Geometry check sheet. Reference: the model listing, model coordinates, mm. A direction names the side the tool comes from. Give positions to 0.01 mm unless a question says otherwise; leave off trailing zeros. Loops run counter-clockwise (first coordinate to the right, second up) from the corner with the lowest first, then second, coordinate; pieces in that order, holes last. Notation, with made-up numbers: (-35.75, 20) - (-28.75, 20) arc R11 ccw to (-28.75, 37) - close; hole circle Ø10 at (5.25, 63). An arc over 180 degrees is marked (long way). Use a Markdown table: item, result. Add a question column.
1. Depth check by flat-ended pin: P1, Ø2.5, axis at x = -16.5, y = -30, coming from the +Z side; P2, Ø6, axis at x = -47.5, y = 0, coming from the -Z side; P3, Ø1, axis at y = -22.5, z = 1, coming from the +X side. Enter the tip coordinate at first touch or a pass-through.
2. Cross-section at B-B on y = -37.5. Enter the section's corners in (x, z), and give its area (3 significant figures).
3. Material ranges on L1, parallel to X at y = -2, z = 1.8; L2, parallel to X at y = 29.5, z = 1.7; L3, parallel to Y at x = 0, z = 1.6, recorded low to high.
4. Cross-section at A-A on x = 47.5. Enter the section's corners in (y, z), and give its area (3 significant figures).
5. Cross-section at C-C on y = -20. Enter the section's corners in (x, z), and give its area (3 significant figures).
6. Draft check along Y on faces 1 (the flat face through (17, -31, 2)), 2 (the cylindrical face through (-11.923, -53.692, 1.479)), 3 (the flat face through (-1, 1, 0)). Enter one of: pulls with the +Y half, pulls with the -Y half, needs draft (parallel to the pull), parting line crosses it, or undercut.
7. Set-up check for faces 4 (the cylindrical face through (45.19, -0.96, 1.48)), 5 (the flat face through (-34, -2, 2)): record each of +Z, -Z, +X, -X, +Y, -Y from which the full face is reachable in a straight line by a thin tool's end or side.
from build123d import *

# Parameters (mm, degrees)
F0_R     = 55
F0_R_2   = 2.5
F0_R_3   = 40
F1_DEPTH = 3
F2_DEPTH = 2


with BuildPart() as f1:
    # F0 (on Top) → F1 (new body)
    with BuildSketch(Plane.XY):
        Circle(F0_R)
        with Locations((-47.5, 0)):
            Circle(F0_R_2, mode=Mode.SUBTRACT)
        Circle(F0_R_3, mode=Mode.SUBTRACT)
        with BuildLine():
            ThreePointArc((50, 0), (47.5, -2.5), (45, 0))
            ThreePointArc((45, 0), (47.5, 2.5), (50, 0))
        make_face(mode=Mode.SUBTRACT)
        Circle(F0_R_3)
        with BuildLine():
            ThreePointArc((19.0424272849, 27.9858618431), (29.3149599181, 16.925), (33.7576809453, 2.4982948569))
            ThreePointArc((33.7576809453, 2.4982948569), (35.584820216, 1.8001107795), (36.35, 0))
            ThreePointArc((36.35, 0), (35.584820216, -1.8001107795), (33.7576809453, -2.4982948569))
            ThreePointArc((33.7576809453, -2.4982948569), (29.3149599181, -16.925), (19.0424272849, -27.9858618431))
            ThreePointArc((19.0424272849, -27.9858618431), (19.3274537677, -28.6234283614), (19.425, -29.3149599181))
            ThreePointArc((19.425, -29.3149599181), (17.5273429883, -31.7413116907), (14.7152536604, -30.4841567))
            ThreePointArc((14.7152536604, -30.4841567), (0, -33.85), (-14.7152536604, -30.4841567))
            ThreePointArc((-14.7152536604, -30.4841567), (-18.175, -31.4800234276), (-19.0424272849, -27.9858618431))
            ThreePointArc((-19.0424272849, -27.9858618431), (-29.3149599181, -16.925), (-33.7576809453, -2.4982948569))
            ThreePointArc((-33.7576809453, -2.4982948569), (-36.35, 0), (-33.7576809453, 2.4982948569))
            ThreePointArc((-33.7576809453, 2.4982948569), (-29.3149599181, 16.925), (-19.0424272849, 27.9858618431))
            ThreePointArc((-19.0424272849, 27.9858618431), (-18.175, 31.4800234276), (-14.7152536604, 30.4841567))
            ThreePointArc((-14.7152536604, 30.4841567), (0, 33.85), (14.7152536604, 30.4841567))
            ThreePointArc((14.7152536604, 30.4841567), (17.5273429883, 31.7413116907), (19.425, 29.3149599181))
            ThreePointArc((19.425, 29.3149599181), (19.3274537677, 28.6234283614), (19.0424272849, 27.9858618431))
        make_face(mode=Mode.SUBTRACT)
        with BuildLine():
            ThreePointArc((33.7576809453, -2.4982948569), (31.35, 0), (33.7576809453, 2.4982948569))
            ThreePointArc((33.7576809453, 2.4982948569), (29.3149599181, 16.925), (19.0424272849, 27.9858618431))
            ThreePointArc((19.0424272849, 27.9858618431), (15.675, 27.1498964086), (14.7152536604, 30.4841567))
            ThreePointArc((14.7152536604, 30.4841567), (0, 33.85), (-14.7152536604, 30.4841567))
            ThreePointArc((-14.7152536604, 30.4841567), (-14.4986482274, 29.9173029064), (-14.425, 29.3149599181))
            ThreePointArc((-14.425, 29.3149599181), (-16.2334684433, 26.9125061504), (-19.0424272849, 27.9858618431))
            ThreePointArc((-19.0424272849, 27.9858618431), (-29.3149599181, 16.925), (-33.7576809453, 2.4982948569))
            ThreePointArc((-33.7576809453, 2.4982948569), (-32.0498892205, 1.734820216), (-31.35, 0))
            ThreePointArc((-31.35, 0), (-32.0498892205, -1.734820216), (-33.7576809453, -2.4982948569))
            ThreePointArc((-33.7576809453, -2.4982948569), (-29.3149599181, -16.925), (-19.0424272849, -27.9858618431))
            ThreePointArc((-19.0424272849, -27.9858618431), (-16.2334684433, -26.9125061504), (-14.425, -29.3149599181))
            ThreePointArc((-14.425, -29.3149599181), (-14.4986482274, -29.9173029064), (-14.7152536604, -30.4841567))
            ThreePointArc((-14.7152536604, -30.4841567), (0, -33.85), (14.7152536604, -30.4841567))
            ThreePointArc((14.7152536604, -30.4841567), (15.675, -27.1498964086), (19.0424272849, -27.9858618431))
            ThreePointArc((19.0424272849, -27.9858618431), (29.3149599181, -16.925), (33.7576809453, -2.4982948569))
        make_face()
    extrude(amount=F1_DEPTH)

    # F0 (on Top) → F2 (join)
    with BuildSketch(Plane.XY):
        with BuildLine():
            ThreePointArc((-14.425, 29.3149599181), (-14.4986482274, 29.9173029064), (-14.7152536604, 30.4841567))
            ThreePointArc((-14.7152536604, 30.4841567), (-15.1641142387, 30.2633795098), (-15.6096633615, 30.0359935701))
            ThreePointArc((-15.6096633615, 30.0359935701), (-15.4718990128, 29.6871124689), (-15.425, 29.3149599181))
            ThreePointArc((-15.425, 29.3149599181), (-16.5207430695, 27.8704612735), (-18.2071017789, 28.5363618006))
            ThreePointArc((-18.2071017789, 28.5363618006), (-18.6267983405, 28.2641979115), (-19.0424272849, 27.9858618431))
            ThreePointArc((-19.0424272849, 27.9858618431), (-16.2334684433, 26.9125061504), (-14.425, 29.3149599181))
        make_face()
        with BuildLine():
            ThreePointArc((-15.6096633615, 30.0359935701), (-15.1641142387, 30.2633795098), (-14.7152536604, 30.4841567))
            ThreePointArc((-14.7152536604, 30.4841567), (-18.175, 31.4800234276), (-19.0424272849, 27.9858618431))
            ThreePointArc((-19.0424272849, 27.9858618431), (-18.6267983405, 28.2641979115), (-18.2071017789, 28.5363618006))
            ThreePointArc((-18.2071017789, 28.5363618006), (-17.675, 30.6139980238), (-15.6096633615, 30.0359935701))
        make_face()
        with BuildLine():
            ThreePointArc((-31.35, 0), (-32.0498892205, 1.734820216), (-33.7576809453, 2.4982948569))
            ThreePointArc((-33.7576809453, 2.4982948569), (-33.7909125792, 1.9991815983), (-33.8167651403, 1.4996317695))
            ThreePointArc((-33.8167651403, 1.4996317695), (-32.7776539063, 1.0488440567), (-32.35, 0))
            ThreePointArc((-32.35, 0), (-32.7776539063, -1.0488440567), (-33.8167651403, -1.4996317695))
            ThreePointArc((-33.8167651403, -1.4996317695), (-33.7909125792, -1.9991815983), (-33.7576809453, -2.4982948569))
            ThreePointArc((-33.7576809453, -2.4982948569), (-32.0498892205, -1.734820216), (-31.35, 0))
        make_face()
        with BuildLine():
            ThreePointArc((-33.8167651403, 1.4996317695), (-33.7909125792, 1.9991815983), (-33.7576809453, 2.4982948569))
            ThreePointArc((-33.7576809453, 2.4982948569), (-36.35, 0), (-33.7576809453, -2.4982948569))
            ThreePointArc((-33.7576809453, -2.4982948569), (-33.7909125792, -1.9991815983), (-33.8167651403, -1.4996317695))
            ThreePointArc((-33.8167651403, -1.4996317695), (-35.35, 0), (-33.8167651403, 1.4996317695))
        make_face()
        with BuildLine():
            ThreePointArc((-15.6096633615, -30.0359935701), (-15.1641142387, -30.2633795098), (-14.7152536604, -30.4841567))
            ThreePointArc((-14.7152536604, -30.4841567), (-14.4986482274, -29.9173029064), (-14.425, -29.3149599181))
            ThreePointArc((-14.425, -29.3149599181), (-16.2334684433, -26.9125061504), (-19.0424272849, -27.9858618431))
            ThreePointArc((-19.0424272849, -27.9858618431), (-18.6267983405, -28.2641979115), (-18.2071017789, -28.5363618006))
            ThreePointArc((-18.2071017789, -28.5363618006), (-16.5207430695, -27.8704612735), (-15.425, -29.3149599181))
            ThreePointArc((-15.425, -29.3149599181), (-15.4718990128, -29.6871124689), (-15.6096633615, -30.0359935701))
        make_face()
        with BuildLine():
            ThreePointArc((-19.0424272849, -27.9858618431), (-18.175, -31.4800234276), (-14.7152536604, -30.4841567))
            ThreePointArc((-14.7152536604, -30.4841567), (-15.1641142387, -30.2633795098), (-15.6096633615, -30.0359935701))
            ThreePointArc((-15.6096633615, -30.0359935701), (-17.675, -30.6139980238), (-18.2071017789, -28.5363618006))
            ThreePointArc((-18.2071017789, -28.5363618006), (-18.6267983405, -28.2641979115), (-19.0424272849, -27.9858618431))
        make_face()
        with BuildLine():
            ThreePointArc((18.2071017789, -28.5363618006), (18.6267983405, -28.2641979115), (19.0424272849, -27.9858618431))
            ThreePointArc((19.0424272849, -27.9858618431), (15.675, -27.1498964086), (14.7152536604, -30.4841567))
            ThreePointArc((14.7152536604, -30.4841567), (15.1641142387, -30.2633795098), (15.6096633615, -30.0359935701))
            ThreePointArc((15.6096633615, -30.0359935701), (16.175, -28.0159218124), (18.2071017789, -28.5363618006))
        make_face()
        with BuildLine():
            ThreePointArc((19.425, -29.3149599181), (19.3274537677, -28.6234283614), (19.0424272849, -27.9858618431))
            ThreePointArc((19.0424272849, -27.9858618431), (18.6267983405, -28.2641979115), (18.2071017789, -28.5363618006))
            ThreePointArc((18.2071017789, -28.5363618006), (18.3694986446, -28.9107029876), (18.425, -29.3149599181))
            ThreePointArc((18.425, -29.3149599181), (17.2971525508, -30.7680609053), (15.6096633615, -30.0359935701))
            ThreePointArc((15.6096633615, -30.0359935701), (15.1641142387, -30.2633795098), (14.7152536604, -30.4841567))
            ThreePointArc((14.7152536604, -30.4841567), (17.5273429883, -31.7413116907), (19.425, -29.3149599181))
        make_face()
        with BuildLine():
            ThreePointArc((33.7576809453, 2.4982948569), (33.7909125792, 1.9991815983), (33.8167651403, 1.4996317695))
            ThreePointArc((33.8167651403, 1.4996317695), (34.8988440567, 1.0723460937), (35.35, 0))
            ThreePointArc((35.35, 0), (34.8988440567, -1.0723460937), (33.8167651403, -1.4996317695))
            ThreePointArc((33.8167651403, -1.4996317695), (33.7909125792, -1.9991815983), (33.7576809453, -2.4982948569))
            ThreePointArc((33.7576809453, -2.4982948569), (35.584820216, -1.8001107795), (36.35, 0))
            ThreePointArc((36.35, 0), (35.584820216, 1.8001107795), (33.7576809453, 2.4982948569))
        make_face()
        with BuildLine():
            ThreePointArc((33.8167651403, -1.4996317695), (32.35, 0), (33.8167651403, 1.4996317695))
            ThreePointArc((33.8167651403, 1.4996317695), (33.7909125792, 1.9991815983), (33.7576809453, 2.4982948569))
            ThreePointArc((33.7576809453, 2.4982948569), (31.35, 0), (33.7576809453, -2.4982948569))
            ThreePointArc((33.7576809453, -2.4982948569), (33.7909125792, -1.9991815983), (33.8167651403, -1.4996317695))
        make_face()
        with BuildLine():
            ThreePointArc((18.2071017789, 28.5363618006), (18.6267983405, 28.2641979115), (19.0424272849, 27.9858618431))
            ThreePointArc((19.0424272849, 27.9858618431), (19.3274537677, 28.6234283614), (19.425, 29.3149599181))
            ThreePointArc((19.425, 29.3149599181), (17.5273429883, 31.7413116907), (14.7152536604, 30.4841567))
            ThreePointArc((14.7152536604, 30.4841567), (15.1641142387, 30.2633795098), (15.6096633615, 30.0359935701))
            ThreePointArc((15.6096633615, 30.0359935701), (17.2971525508, 30.7680609053), (18.425, 29.3149599181))
            ThreePointArc((18.425, 29.3149599181), (18.3694986446, 28.9107029876), (18.2071017789, 28.5363618006))
        make_face()
        with BuildLine():
            ThreePointArc((14.7152536604, 30.4841567), (15.675, 27.1498964086), (19.0424272849, 27.9858618431))
            ThreePointArc((19.0424272849, 27.9858618431), (18.6267983405, 28.2641979115), (18.2071017789, 28.5363618006))
            ThreePointArc((18.2071017789, 28.5363618006), (16.175, 28.0159218124), (15.6096633615, 30.0359935701))
            ThreePointArc((15.6096633615, 30.0359935701), (15.1641142387, 30.2633795098), (14.7152536604, 30.4841567))
        make_face()
    extrude(amount=F2_DEPTH)


solid = f1.part
Values found:
| question | item | result |
|---|---|---|
| 1 | P1 | stops at z = 2 |
| 1 | P2 | stops at z = 0 |
| 1 | P3 | stops at x = 50.41 |
| 2 | outline | (-40.23, 0) - (40.23, 0) - (40.23, 3) - (-40.23, 3) - close |
| 2 | area | 241 mm2 |
| 3 | L1 | x = -54.96 to -49, -46 to 46, 49 to 54.96 |
| 3 | L2 | x = -46.42 to -18.41, -15.44 to 15.44, 18.41 to 46.42 |
| 3 | L3 | y = -55 to 55 |
| 4 | outline | (-27.73, 0) - (-2.5, 0) - (-2.5, 3) - (-27.73, 3) - close; (2.5, 0) - (27.73, 0) - (27.73, 3) - (2.5, 3) - close |
| 4 | area | 151 mm2 |
| 5 | outline | (-51.23, 0) - (51.23, 0) - (51.23, 3) - (-51.23, 3) - close |
| 5 | area | 307 mm2 |
| 6 | face 1 | undercut |
| 6 | face 2 | parting line crosses it |
| 6 | face 3 | needs draft |
| 7 | face 4 | +Z, -Z |
| 7 | face 5 | +Z |
